Part print with two shaded views. Sizes in mm from the minimum x, y, z corner. A direction names the side the tool comes from. Round coordinates to 2 decimals unless told otherwise and drop trailing zeros. Loops run counter-clockwise (first coordinate to the right, second up) from the corner with the lowest first, then second, coordinate; pieces in that order, holes last. Notation, with made-up numbers: M 11.25,57 L 49.25,57 A36 cw 49.25,93 Z; hole C -18.5,86.5 d3. An arc over 180 degrees is marked long. Use a Markdown table: item, result. Add a question column.
Item 1: Saw through at D-D on y = 3. Write the cut outline in (x, z), then the cut area to 3 significant figures.
Item 2: Saw through at B-B on z = 5.5. Write the cut outline in (x, y).
Item 3: Pin check, flat tips, straight feed: P1, Ø3.5, axis at x = 15, y = 7, coming from the -Z side; P2, Ø2.5, axis at x = 31, y = 7, coming from the -Z side. Stop position of each tip, or through.
Item 4: Saw through at A-A on y = 7. Write the cut outline in (x, z), then the cut area to 3 significant figures.
Item 5: Saw through at C-C on x = 15. Write the cut outline in (y, z).
Item 6: Two-plate mould, pull along X, no slides. Class the marked faces 3, 4, 5 and 6: +X half, -X half, draft (parallel to the pull), parting line (faces both ways), or undercut.
Item 7: Tool access for the marked faces 1 and 2: list every direction of +Z, -Z, +X, -X, +Y, -Y with a clear straight run to the whole face (end or side of a thin tool).
Item 8: Wall check: L1, parallel to Y at x = 15, z = 5.55; L2, parallel to X at y = 9.25, z = 5.75; L3, parallel to X at y = 6.5, z = 6.25. Give the ranges that are in metal, low to high. Write a range as from..to.
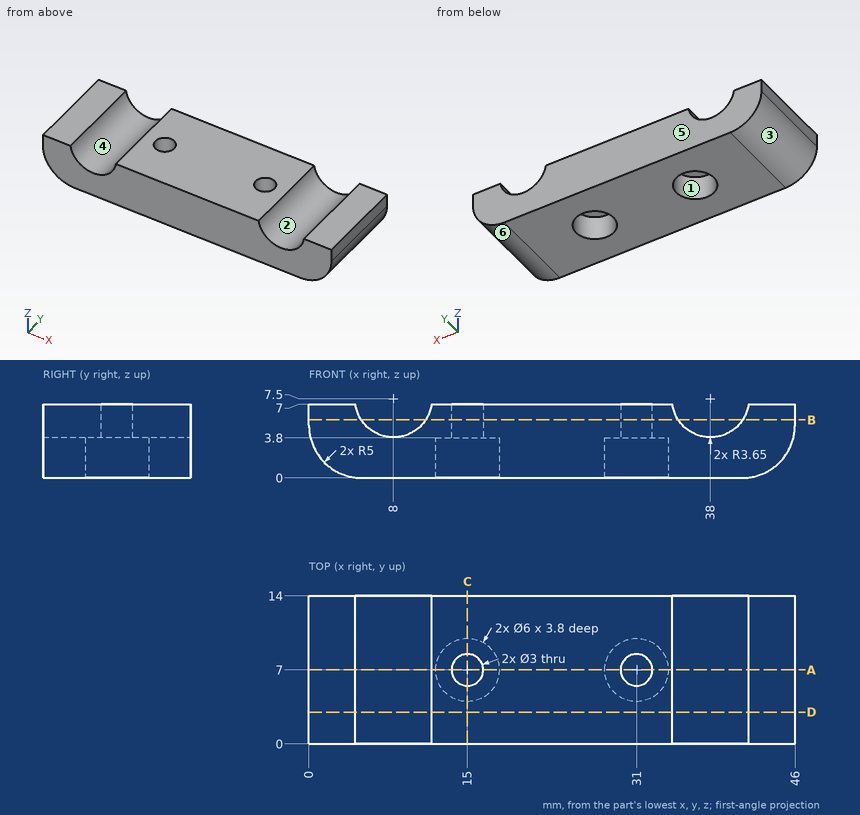
Entries:
| question | item | result |
|---|---|---|
| 1 | outline | M 0,5 A5 ccw 5,0 L 41,0 A5 ccw 46,5 L 46,7 L 41.62,7 A3.65 cw 34.38,7 L 11.62,7 A3.65 cw 4.38,7 L 0,7 Z |
| 1 | area | 277 mm2 |
| 2 | outline | M 0,0 L 4.95,0 L 4.95,14 L 0,14 Z; M 11.05,0 L 34.95,0 L 34.95,14 L 11.05,14 Z; M 41.05,0 L 46,0 L 46,14 L 41.05,14 Z; hole C 15,7 d3; hole C 31,7 d3 |
| 3 | P1 | z = 3.8 |
| 3 | P2 | through |
| 4 | outline | M 0,5 A5 ccw 5,0 L 12,0 L 12,3.8 L 13.5,3.8 L 13.5,7 L 11.62,7 A3.65 cw 4.38,7 L 0,7 Z; M 16.5,3.8 L 18,3.8 L 18,0 L 28,0 L 28,3.8 L 29.5,3.8 L 29.5,7 L 16.5,7 Z; M 32.5,3.8 L 34,3.8 L 34,0 L 41,0 A5 ccw 46,5 L 46,7 L 41.62,7 A3.65 cw 34.38,7 L 32.5,7 Z |
| 4 | area | 212 mm2 |
| 5 | outline | M 0,0 L 4,0 L 4,3.8 L 5.5,3.8 L 5.5,7 L 0,7 Z; M 8.5,3.8 L 10,3.8 L 10,0 L 14,0 L 14,7 L 8.5,7 Z |
| 6 | face 3 | -X half |
| 6 | face 4 | undercut |
| 6 | face 5 | draft |
| 6 | face 6 | +X half |
| 7 | face 1 | -Z |
| 7 | face 2 | +Z, +Y, -Y |
| 8 | L1 | 0..5.5, 8.5..14 |
| 8 | L2 | 0..4.8, 11.2..34.8, 41.2..46 |
| 8 | L3 | 0..4.57, 11.43..13.59, 16.41..29.59, 32.41..34.57, 41.43..46 |
